```python
from build123d import *

# Parameters (mm, degrees)
F0_W     = 50
F0_H     = 50
F1_DEPTH = 10
F4_D     = 16
F5_T     = -3
F6_R     = 5


with BuildPart() as f1:
    # F0 (on Top) → F1 (new body)
    with BuildSketch(Plane.XY):
        Rectangle(F0_W, F0_H)
    extrude(amount=F1_DEPTH)

    # F4 (through all)
    with Locations(Plane.XY.offset(10)):
        with Locations((0, 0)):
            Hole(F4_D / 2)

    # F5
    f5_openings = [f1.faces().sort_by_distance(p)[0] for p in [
        (24.292893, 0, 10),
    ]]
    offset(amount=F5_T, openings=f5_openings)

    # F6
    f6_edges = [f1.edges().sort_by_distance(p)[0] for p in [
        (-25, 0, 0),
        (0, 25, 0),
        (25, 0, 0),
        (0, -25, 0),
    ]]
    fillet(f6_edges, radius=F6_R)


solid = f1.part
```
Part model, mm, in its own coordinate system. A direction names the side the tool comes from. Round coordinates to 2 decimals unless told otherwise and drop trailing zeros. Order: outer loops, then holes, each group sorted by start corner. A loop starts at its lowest first (then second) coordinate and runs counter-clockwise, first axis right, second up. Notation, with made-up numbers: M 70,57 L 94,57 A12 cw 94,79 Z; hole C 9,-34.75 d3. An arc over 180 degrees is marked long. Put each result on its own line as item: value. Start each with the question number.
1. Drill centre lines: probe 1 along Y at (x, z) = (0, 7); probe 2 along Y at (x, z) = (-4, 7); probe 3 along X at (y, z) = (8.5, 6). Where is each one in solid material? Low to high. Write a range as [from, to].
2. Two-plate mould, pull along X, no slides. Class faces 1 (the face through (-24, 0, 2)), 2 (the face through (0, -25, 7)), 3 (the face through (22, 0, 6)): +X half, -X half, draft (parallel to the pull), parting line (faces both ways), or undercut.
3. Slice it at B-B on y = 0. List the corners of the cut face in (x, z), then the cut area to 3 significant figures.
4. Drop a flat-ended pin along its axis: pin 1 (1.5 mm diameter, centred on y = 7, z = 2, fed in from -X). Give the stop position or say it passes through.
5. Tool access for faces 4 (the face through (23, 0, 1)), 5 (the face through (0, -22, 6)): list every direction of +Z, -Z, +X, -X, +Y, -Y with a clear straight run to the whole face (end or side of a thin tool).
6. Slice it at D-D on z = 1. List the corners of the cut face in (x, y), then the cut area to 3 significant figures.
7. Slice it at A-A on z = 8. List the corners of the cut face in (x, y).
Findings:
1. probe 1: [-25, -22], [-11, -8], [8, 11], [22, 25]
1. probe 2: [-25, -22], [-10.25, -6.93], [6.93, 10.25], [22, 25]
1. probe 3: [-25, -22], [-6.98, 6.98], [22, 25]
2. face 1: -X half
2. face 2: draft
2. face 3: undercut
3. outline: M -25,5 A5 ccw -20,0 L -8,0 L -8,10 L -11,10 L -11,3 L -22,3 L -22,10 L -25,10 Z; M 8,0 L 20,0 A5 ccw 25,5 L 25,10 L 22,10 L 22,3 L 11,3 L 11,10 L 8,10 Z
3. area: 175 mm2
4. pin 1: x = -24.47
5. face 4: -Z, +X, +Y, -Y
5. face 5: +Z
6. outline: M -23,-23 L 23,-23 L 23,23 L -23,23 Z; hole C 0,0 d16
6. area: 1,910 mm2
7. outline: M -25,-25 L 25,-25 L 25,25 L -25,25 Z; C 0,0 d22; hole M -22,-22 L 22,-22 L 22,22 L -22,22 Z; hole C 0,0 d16
